```python
from build123d import *

# Parameters (mm, degrees)
SKETCH_1_W          = 13.5
SKETCH_1_H          = 25
SKETCH_1_R          = 1.7
SKETCH_1_W_2        = 2.5
SKETCH_1_H_2        = 4.75
EXTRUDE_1_DEPTH     = 1.2
SKETCH_2_R          = 2.1
EXTRUDE_2_DEPTH     = 15.5
SKETCH_3_R          = 1.5
CUT_EXTRUDE_1_DEPTH = 18
SKETCH_4_W          = 4.6
SKETCH_4_H          = 6
CUT_EXTRUDE_2_DEPTH = 5


with BuildPart() as part:
    # 草图1 → 凸台-拉伸1 (new body)
    # profile 1 of 3: a face of its own
    with BuildSketch(Plane.XY):
        Rectangle(SKETCH_1_W, SKETCH_1_H)
        with Locations((-1.75, -7)):
            Circle(SKETCH_1_R, mode=Mode.SUBTRACT)
        with Locations((-1.75, 7)):
            Circle(SKETCH_1_R, mode=Mode.SUBTRACT)
    # profile 2 of 3: a face of its own
    with BuildSketch(Plane.XY):
        with Locations((8, 5.375)):
            Rectangle(SKETCH_1_W_2, SKETCH_1_H_2)
    # profile 3 of 3: a face of its own
    with BuildSketch(Plane.XY):
        with Locations((8, -5.375)):
            Rectangle(SKETCH_1_W_2, SKETCH_1_H_2)
    extrude(amount=EXTRUDE_1_DEPTH)

    # 草图2 → 凸台-拉伸2 (add)
    with BuildSketch(Plane.XZ.offset(7.75)):
        with Locations(Location((9.25, 2.1, 0), (0, 0, 270))):
            Circle(SKETCH_2_R)
    extrude(amount=-EXTRUDE_2_DEPTH)

    # 草图3 → 切除-拉伸1 (cut)
    with BuildSketch(Plane.XZ.offset(7.75)):
        with Locations(Location((9.25, 2.1, 0), (0, 0, 270))):
            Circle(SKETCH_3_R)
    extrude(amount=-CUT_EXTRUDE_1_DEPTH, mode=Mode.SUBTRACT)

    # 草图4 → 切除-拉伸2 (cut, symmetric)
    with BuildSketch(Plane.XY.offset(1.2)):
        with Locations((9.05, 0)):
            Rectangle(SKETCH_4_W, SKETCH_4_H)
    extrude(amount=CUT_EXTRUDE_2_DEPTH, both=True, mode=Mode.SUBTRACT)


solid = part.part
```
Read the model definition and answer for the solid it produces. Units are mm, in the model's axes. A direction names the side the tool comes from. Give positions to 0.01 mm unless a question says otherwise; leave off trailing zeros. Write each loop counter-clockwise with the first axis right and the second up, starting at its lowest first coordinate (ties: lowest second). Pieces come first, ordered by that corner, then holes. Notation, with made-up numbers: (0, -19.5) - (45, -19.5) arc R29 cw to (45, 15.5) - close; hole circle Ø7 at (38, 29.25). An arc over 180 degrees is marked (long way). Write item = value, one per line. Start each with the question number.
Item 1: The mould has two halves that part along X. Classify faces 5 (the flat face through (6.75, 10, 1)), 6 (the flat face through (1, 0, 0)), 7 (the cylindrical face through (-0.97, -8.51, 0.59)), 8 (the cylindrical face through (7.786, -5.408, 2.425)): +X half, -X half, draft (parallel to the pull), parting line (faces both ways), or undercut.
Item 2: Find section B-B (x = -1.75). Give the vertices of the cut face in (y, z), then the cut area to 3 significant figures.
Item 3: Find the intervals of material crossed by probe 1 along Y at (x, z) = (-1.75, 0.55); probe 2 along X at (y, z) = (-4.85, 2.1); probe 3 along Z at (x, y) = (-3.25, 6), in increasing order. Write a range as [from, to].
Item 4: Find section A-A (y = -7). Give the vertices of the cut face in (x, z), then the cut area to 3 significant figures.
Item 5: Find section C-C (z = 3.05). Give the vertices of the cut face in (x, y), then the cut area to 3 significant figures.
Item 6: A tool of negligible diameter and unlimited length cuts with its end or side. For faces 1 (the flat face through (7.5, 7.75, 1.7)), 2 (the flat face through (6.75, 0, 1)), 3 (the flat face through (7.5, -7.75, 1.7)), 4 (the cylindrical face through (-0.97, 5.49, 0.59)), from which of +Z, -Z, +X, -X, +Y, -Y can it reach the whole face along a straight path? Write none if from no direction.
Item 7: Each of these flat-tipped pins is pushed along its axis until it touches: P1, Ø5.5, axis at x = -1.75, y = 7, coming from the +Z side; P2, Ø1, axis at y = -9.5, z = 0.5, coming from the +X side; P3, Ø1.5, axis at x = 4.5, z = 3.5, coming from the -Y side; P4, Ø1.3, axis at x = 8, z = 3, coming from the -Y side. Where does it stop, or does it pass through?
Item 8: Find section D-D (x = 9). Give the vertices of the cut face in (y, z), then the cut area to 3 significant figures.
Response:
q1.face_5 = +X half
q1.face_6 = draft
q1.face_7 = undercut
q1.face_8 = undercut
q2.outline = (-12.5, 0) - (-8.7, 0) - (-8.7, 1.2) - (-12.5, 1.2) - close; (-5.3, 0) - (5.3, 0) - (5.3, 1.2) - (-5.3, 1.2) - close; (8.7, 0) - (12.5, 0) - (12.5, 1.2) - (8.7, 1.2) - close
q2.area = 21.8 mm²
q3.probe_1 = [-12.5, -8.7], [-5.3, 5.3], [8.7, 12.5]
q3.probe_2 = [7.15, 7.75], [10.75, 11.35]
q3.probe_3 = [0, 1.2]
q4.outline = (-6.75, 0) - (-3.45, 0) - (-3.45, 1.2) - (-6.75, 1.2) - close; (-0.05, 0) - (9.25, 0) arc R2.1 ccw (long way) to (7.35, 1.2) - (-0.05, 1.2) - close; hole circle Ø3 at (9.25, 2.1)
q4.area = 20.3 mm²
q5.outline = (7.38, -7.75) - (8.09, -7.75) - (8.09, -3) - (7.38, -3) - close; (7.38, 3) - (8.09, 3) - (8.09, 7.75) - (7.38, 7.75) - close; (10.41, -7.75) - (11.12, -7.75) - (11.12, -3) - (10.41, -3) - close; (10.41, 3) - (11.12, 3) - (11.12, 7.75) - (10.41, 7.75) - close
q5.area = 13.5 mm²
q6.face_1 = +Z, -Z, +X, +Y
q6.face_2 = +Z, -Z, +X
q6.face_3 = +Z, -Z, +X, -Y
q6.face_4 = +Z, -Z
q7.P1 = 1.2
q7.P2 = 6.75
q7.P3 = through
q7.P4 = -7.75
q8.outline = (-7.75, 0) - (-3, 0) - (-3, 0.62) - (-7.75, 0.62) - close; (-7.75, 3.58) - (-3, 3.58) - (-3, 4.19) - (-7.75, 4.19) - close; (3, 0) - (7.75, 0) - (7.75, 0.62) - (3, 0.62) - close; (3, 3.58) - (7.75, 3.58) - (7.75, 4.19) - (3, 4.19) - close
q8.area = 11.7 mm²
